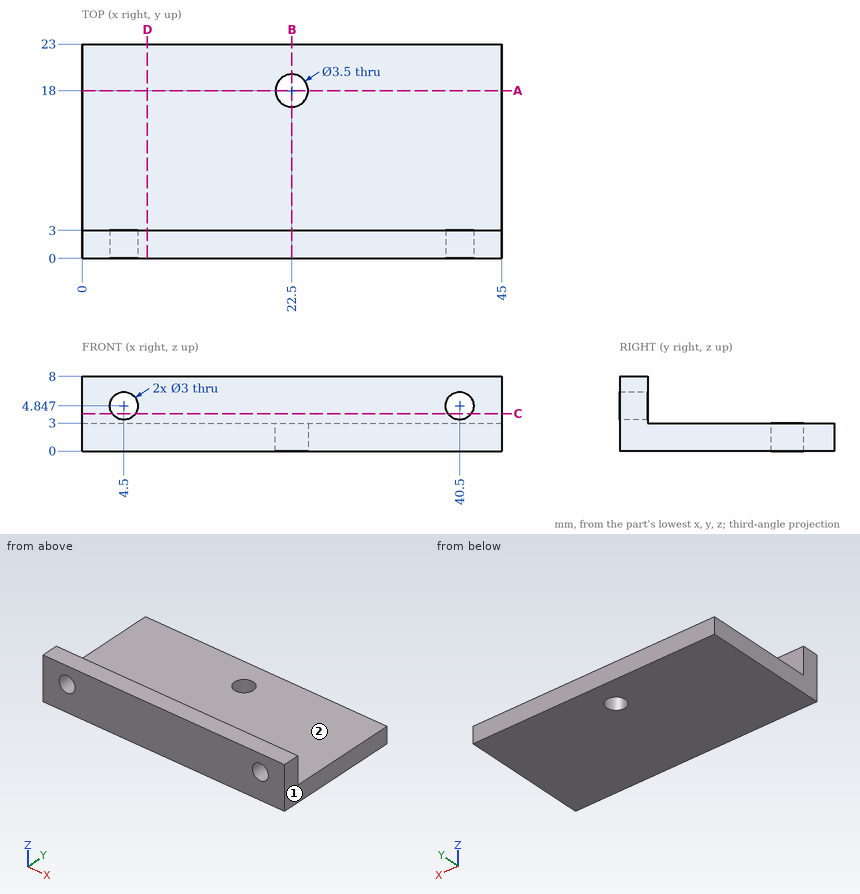
Geometry: see drawing. Coordinates: mm, zero at the bounding-box minimum. A direction names the side the tool comes from. Give positions to 0.01 mm unless a question says otherwise; leave off trailing zeros. Loops run counter-clockwise (first coordinate to the right, second up) from the corner with the lowest first, then second, coordinate; pieces in that order, holes last. Notation, with made-up numbers: (-8, 34) - (14, 34) arc R8 ccw to (14, 47) - close; hole circle Ø3 at (70.5, -23.5). An arc over 180 degrees is marked (long way). One line per question, with ' | ' between items. Start each with the question number.
(1) Section query C-C on z = 4. Return loops of the section in (x, y), then the cut area to 3 significant figures.
(2) Contact query for flat-ended pins moving along their axis: pin 1 (4 mm diameter, centred on x = 26, z = 4.5, fed in from -Y); pin 2 (2.5 mm diameter, centred on x = 40.5, z = 4.85, fed in from +Y); pin 3 (1.5 mm diameter, centred on x = 19, z = 4.5, fed in from +Y); pin 4 (6 mm diameter, centred on x = 12.5, y = 7, fed in from +Z). Output: stop coordinate, or through.
(3) Reachability of the marked faces 1 and 2 from +Z, -Z, +X, -X, +Y, -Y: full face, straight path, thin tool, end or side. Return the list, or none.
(4) Section query B-B on x = 22.5. Return loops of the section in (y, z).
(5) Ray query, line 1 (Y direction, x = 22.5, z = 1.95); line 2 (X direction, y = 1, z = 4); line 3 (Z direction, x = 28, y = 16.75). Return the intervals inside material, ascending. Write a range as from..to.
(6) Section query D-D on x = 7. Return loops of the section in (y, z), then the cut area to 3 significant figures.
(7) Section query A-A on y = 18. Return loops of the section in (x, z).
The answers:
1) outline: (0, 0) - (3.26, 0) - (3.26, 3) - (0, 3) - close; (5.74, 0) - (39.26, 0) - (39.26, 3) - (5.74, 3) - close; (41.74, 0) - (45, 0) - (45, 3) - (41.74, 3) - close | area: 120 mm2
2) pin 1: y = 0 | pin 2: through | pin 3: y = 3 | pin 4: z = 3
3) face 1: +Z, -Z, +X, +Y, -Y | face 2: +Z, +X, -X, +Y
4) outline: (0, 0) - (16.25, 0) - (16.25, 3) - (3, 3) - (3, 8) - (0, 8) - close; (19.75, 0) - (23, 0) - (23, 3) - (19.75, 3) - close
5) line 1: 0..16.25, 19.75..23 | line 2: 0..3.26, 5.74..39.26, 41.74..45 | line 3: 0..3
6) outline: (0, 0) - (23, 0) - (23, 3) - (3, 3) - (3, 8) - (0, 8) - close | area: 84.0 mm2
7) outline: (0, 0) - (20.75, 0) - (20.75, 3) - (0, 3) - close; (24.25, 0) - (45, 0) - (45, 3) - (24.25, 3) - close
